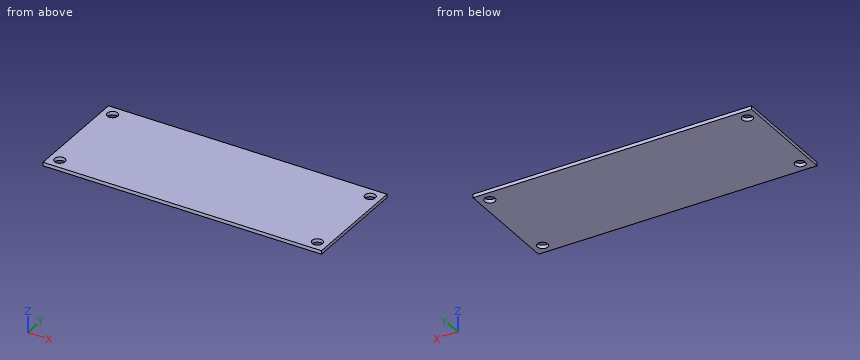
Autodesk Fusion 360 part; units mm, degrees
sketch "スケッチ1" plane through (0, 0, 0) normal (0, 0, 1) x (1, 0, 0)
  line L0 (0, 0) -> (80, 0)
  line L1 (80, 0) -> (80, 31)
  line L2 (80, 31) -> (0, 31)
  line L3 (0, 31) -> (0, 0)
  line L4 (0, 31) -> (3, 31)
  line L5 (0, 28) -> (0, 31)
  circle A0 centre (3, 28) radius 1.5
  line L6 (0, 0) -> (3, 0)
  line L7 (0, 3) -> (0, 0)
  circle A1 centre (3, 3) radius 1.5
  line L8 (80, 0) -> (77, 0)
  line L9 (80, 3) -> (80, 0)
  line L10 (80, 31) -> (77, 31)
  line L11 (80, 28) -> (80, 31)
  circle A2 centre (77, 28) radius 1.5
  circle A3 centre (77, 3) radius 1.5
  dimension "d1" = 80
  dimension "d2" = 31
  dimension "d3" = 3
  dimension "d4" = 3
  dimension "d5" = 3
  dimension "d6" = 3
  dimension "d7" = 3
  dimension "d8" = 3
  dimension "d9" = 3
extrude "押し出し1" add sketch "スケッチ1" along normal blind 1
The model under review builds one solid part; all positions refer to its coordinate system, in mm. Round coordinates to 2 decimals unless told otherwise and drop trailing zeros. Loops run counter-clockwise (first coordinate to the right, second up) from the corner with the lowest first, then second, coordinate; pieces in that order, holes last. Notation, with made-up numbers: (-23.75, 14.25) -> (17.25, 14.25) arc R7 cw to (17.25, 24.25) -> close; hole circle Ø11 at (-31.75, 79.5). An arc over 180 degrees is marked (long way). Answer in a Markdown table with one row per item.
1) Wall thickness on line 1 along Y through (x, z) = (77, 0.75); line 2 along Y through (x, z) = (76.5, 0.5); line 3 along X through (y, z) = (3.5, 0.35): over which ranges is each line inside the solid? List them lowest first.
Taken from the geometry:
| item | result |
|---|---|
| line 1 | y = 0 to 1.5, 4.5 to 26.5, 29.5 to 31 |
| line 2 | y = 0 to 1.59, 4.41 to 26.59, 29.41 to 31 |
| line 3 | x = 0 to 1.59, 4.41 to 75.59, 78.41 to 80 |
2) Consider section A-A, the plane x = 77. Write out the cut boundary in (y, z).
Taken from the geometry:
| item | result |
|---|---|
| outline | (0, 0) -> (1.5, 0) -> (1.5, 1) -> (0, 1) -> close; (4.5, 0) -> (26.5, 0) -> (26.5, 1) -> (4.5, 1) -> close; (29.5, 0) -> (31, 0) -> (31, 1) -> (29.5, 1) -> close |
3) Consider section B-B, the plane y = 28. Write out the cut boundary in (x, z), plus the area to 3 significant figures.
Taken from the geometry:
| item | result |
|---|---|
| outline | (0, 0) -> (1.5, 0) -> (1.5, 1) -> (0, 1) -> close; (4.5, 0) -> (75.5, 0) -> (75.5, 1) -> (4.5, 1) -> close; (78.5, 0) -> (80, 0) -> (80, 1) -> (78.5, 1) -> close |
| area | 74.0 mm² |
